```python
from build123d import *

# Parameters (mm, degrees)
F0_W     = 400
F0_H     = 400
F1_DEPTH = 40
F2_W     = 40
F2_H     = 40
F3_DEPTH = 360
F4_R     = 23.11
F5_R     = 5
F6_R     = 5


with BuildPart() as f1:
    # F0 (on Top) → F1 (new body)
    with BuildSketch(Plane.XY):
        with Locations((-9.5043759793, 29.5748232458)):
            Rectangle(F0_W, F0_H)
    extrude(amount=F1_DEPTH)

    # F2 (on face) → F3 (join)
    with BuildSketch(Plane.XY.offset(40)):
        with Locations((130.4956240207, -110.4251767542)):
            Rectangle(F2_W, F2_H)
        with Locations((-149.5043759793, -110.4251767542)):
            Rectangle(F2_W, F2_H)
        with Locations((-149.5043759793, 169.5748232458)):
            Rectangle(F2_W, F2_H)
        with Locations((130.4956240207, 169.5748232458)):
            Rectangle(F2_W, F2_H)
    extrude(amount=F3_DEPTH)

    # F4
    f4_edges = [f1.edges().sort_by_distance(p)[0] for p in [
        (-209.504376, 29.574823, 0),
        (-9.504376, 229.574823, 0),
        (-9.504376, -170.425177, 0),
        (190.495624, 29.574823, 0),
    ]]
    fillet(f4_edges, radius=F4_R)

    # F5
    f5_edges = [f1.edges().sort_by_distance(p)[0] for p in [
        (-129.504376, 189.574823, 220),
        (-129.504376, 149.574823, 220),
        (-169.504376, -130.425177, 220),
        (-129.504376, -130.425177, 220),
        (-129.504376, -90.425177, 220),
        (-169.504376, -90.425177, 220),
        (-169.504376, 189.574823, 220),
        (-169.504376, 149.574823, 220),
    ]]
    fillet(f5_edges, radius=F5_R)

    # F6
    f6_edges = [f1.edges().sort_by_distance(p)[0] for p in [
        (150.495624, -130.425177, 220),
        (150.495624, -90.425177, 220),
        (150.495624, 149.574823, 220),
        (150.495624, 189.574823, 220),
        (110.495624, 189.574823, 220),
        (110.495624, 149.574823, 220),
        (110.495624, 169.574823, 40),
        (110.495624, 169.574823, 400),
        (110.495624, -90.425177, 220),
        (110.495624, -130.425177, 220),
        (130.495624, 189.574823, 40),
        (130.495624, 149.574823, 40),
        (150.495624, 169.574823, 40),
    ]]
    fillet(f6_edges, radius=F6_R)


solid = f1.part
```
For this review, take the finished solid that the model builds, in its own axes (mm). A direction names the side the tool comes from. Round coordinates to 2 decimals unless told otherwise and drop trailing zeros. Write each loop counter-clockwise with the first axis right and the second up, starting at its lowest first coordinate (ties: lowest second). Pieces come first, ordered by that corner, then holes. Notation, with made-up numbers: (-35.75, 29.25) -> (19.25, 29.25) arc R31 cw to (19.25, 63.25) -> close; hole circle Ø3 at (62, -17). An arc over 180 degrees is marked (long way). One line per question, with ' | ' between items. Start each with the question number.
(1) Add section A-A, the plane z = 52. Give the number of separate pieces and of enclosed holes in the cut face, plus the area to 3 significant figures.
(2) Mouldability with a two-part tool opening along Y and no side actions: class faces 5 (the face through (130, 189.575, 220)), 6 (the face through (130, 149.575, 220)), 7 (the face through (-202.914, 32.375, 6.949)) as released by +Y, released by -Y, zero draft, split by the parting line, or undercut.
(3) Add section C-C, the plane y = 59. Write out the cut boundary in (x, z), plus the area to 3 significant figures.
(4) Tool access review of faces 1 (the face through (-12, 32, 40)), 2 (the face through (110.496, 169, 218)), 3 (the face through (-150, 149.575, 217)), 4 (the face through (-169.504, -111, 217)): name each direction out of +Z, -Z, +X, -X, +Y, -Y from which nothing blocks a thin tool from reaching the whole face with its end or side.
(5) For line 1 along X through (y, z) = (-103.5, 234); line 2 along Z through (x, y) = (101.5, -88); line 3 along Y through (x, z) = (-167, 187.5), list the stretches that pass through material, from the lowest coordinate up. Write a range as from..to.
(6) Add section D-D, the plane x = 134. Write out the cut boundary in (y, z).
(7) Add section B-B, the plane x = -66.5. Write out the cut boundary in (y, z), plus the area to 3 significant figures.
(8) Insertion check: P1, Ø24, axis at x = 123.5, z = 298, coming from the -Y side; P2, Ø15, axis at y = -106, z = 171, coming from the -X side; P3, Ø15, axis at y = -117.5, z = 167, coming from the +X side. Each pin has a flat end and moves straight along its axis. Give the tip position at first contact, or say it passes through.
Answer list:
1) separate pieces: 4 | enclosed holes: 0 | area: 6,310 mm²
2) face 5: released by +Y | face 6: undercut | face 7: zero draft
3) outline: (-209.5, 23.11) arc R23.11 ccw to (-186.39, 0) -> (167.39, 0) arc R23.11 ccw to (190.5, 23.11) -> (190.5, 40) -> (-209.5, 40) -> close | area: 15,800 mm²
4) face 1: +Z | face 2: +Z, +Y, -Y | face 3: +Z, +X, -X | face 4: +Z, -X, +Y, -Y
5) line 1: -169.5..-129.5, 110.5..150.5 | line 2: 0..40 | line 3: -129.76..-91.09, 150.24..188.91
6) outline: (-170.43, 23.11) arc R23.11 ccw to (-147.32, 0) -> (206.46, 0) arc R23.11 ccw to (229.57, 23.11) -> (229.57, 40) -> (194.57, 40) arc R5 cw to (189.57, 45) -> (189.57, 400) -> (149.57, 400) -> (149.57, 45) arc R5 cw to (144.57, 40) -> (-90.43, 40) -> (-90.43, 400) -> (-130.43, 400) -> (-130.43, 40) -> (-170.43, 40) -> close
7) outline: (-170.43, 23.11) arc R23.11 ccw to (-147.32, 0) -> (206.46, 0) arc R23.11 ccw to (229.57, 23.11) -> (229.57, 40) -> (-170.43, 40) -> close | area: 15,800 mm²
8) P1: y = -130.43 | P2: x = -169.5 | P3: x = 150.5
